from build123d import *

# Parameters (mm, degrees)
F0_R     = 26.289
F0_R_2   = 5.207
F1_DEPTH = 15.24
F2_R     = 28.829
F2_R_2   = 5.207
F3_DEPTH = 2.54
F5_DEPTH = 17.781
F6_COUNT = 3
F6_ANGLE = 240
F8_SIZE2 = 1.27
F8_SIZE  = 0.3402954744


with BuildPart() as f1:
    # F0 (on Right) → F1 (new body)
    with BuildSketch(Plane.YZ):
        Circle(F0_R)
        Circle(F0_R_2, mode=Mode.SUBTRACT)
    extrude(amount=-F1_DEPTH)

    # F2 (on face) → F3 (join)
    with BuildSketch(Plane.YZ):
        Circle(F2_R)
        Circle(F2_R_2, mode=Mode.SUBTRACT)
    extrude(amount=F3_DEPTH)


with BuildPart() as f5:
    # F4 (on face) → F5 (new body, through all)
    with BuildSketch(Plane(origin=(-15.24, 0, 0), x_dir=(0, -1, 0), z_dir=(-1, 0, 0))):
        with BuildLine():
            ThreePointArc((-28.3910227116, -5.006103314), (-23.5858740231, -39.2113912621), (8.8826653964, -27.4264379104))
            add(Edge.make_bspline(
                [(8.8826653964, -27.4264379104), (8.6161177773, -26.6034358722), (8.3394760096, -25.8031213114), (8.0525136679, -25.025358032)],
                knots=[0, 0, 0, 0, 1.8877220202, 1.8877220202, 1.8877220202, 1.8877220202], degree=3))
            ThreePointArc((8.0525136679, -25.025358032), (-13.5505111701, -22.527653407), (-25.8808899077, -4.6142235084))
            add(Edge.make_bspline(
                [(-25.8808899077, -4.6142235084), (-26.7024403228, -4.7252100836), (-27.5390757823, -4.8558820842), (-28.3910227116, -5.006103314)],
                knots=[41.6093954543, 41.6093954543, 41.6093954543, 41.6093954543, 43.4971174745, 43.4971174745, 43.4971174745, 43.4971174745], degree=3))
        make_face()
        with BuildLine():
            ThreePointArc((-25.8808899077, -4.6142235084), (-13.5505111701, -22.527653407), (8.0525136679, -25.025358032))
            add(Edge.make_bspline(
                [(8.0525136679, -25.025358032), (2.0142176142, -8.6595697091), (-8.5937274184, -2.2788306654), (-25.8808899077, -4.6142235084)],
                knots=[1.8877220202, 1.8877220202, 1.8877220202, 1.8877220202, 41.6093954543, 41.6093954543, 41.6093954543, 41.6093954543], degree=3))
        make_face()
    extrude(amount=-F5_DEPTH)


with BuildPart() as f6_1:
    # F6: instance of F5
    add(f5.part.rotate(Axis((0, 0, 0), (1, 0, 0)), 1 * F6_ANGLE / (F6_COUNT - 1)))


with BuildPart() as f6_2:
    # F6: instance of F5
    add(f5.part.rotate(Axis((0, 0, 0), (1, 0, 0)), 2 * F6_ANGLE / (F6_COUNT - 1)))


with BuildPart() as f1_1:
    add(f1.part)

    # F7: cut F5, F6_2, F6_1
    add(f5.part, mode=Mode.SUBTRACT)
    add(f6_2.part, mode=Mode.SUBTRACT)
    add(f6_1.part, mode=Mode.SUBTRACT)

    # F8
    f8_edges = [f1_1.edges().sort_by_distance(p)[0] for p in [
        (-15.24, 26.284776, 0.47126),
        (-15.24, -13.550511, 22.527653),
        (-15.24, -12.734265, -22.998914),
    ]]
    f8_side = f1_1.faces().sort_by_distance((-15.24, 4.091505, 7.389523))[0]
    chamfer(f8_edges, length=F8_SIZE, length2=F8_SIZE2, reference=f8_side)


solid = f1_1.part
Could you check a few things on this model? Use its own coordinates, in mm. A direction names the side the tool comes from. Coordinates: 2 decimals unless noted, no trailing zeros.
1. For faces 1 (the face through (1.3, -14, -25.2)), 2 (the face through (-6.887, -12.797, -22.964)), 3 (the face through (-6.887, -13.489, 22.564)), 4 (the face through (-6.887, 26.286, 0.4)), which set-ups out of +Z, -Z, +X, -X, +Y, -Y let a thin tool reach every point of the face, with its end or its side?
2. I need wall thicknesses on L1, parallel to Z at x = -10.5, y = 0; L2, parallel to Z at x = -13.5, y = -2; L3, parallel to Z at x = -14.25, y = 19. Which ranges of each line are inside material? Lowest first, please.
3. For P1, Ø2, axis at x = -8, y = 22, coming from the -Z side; P2, Ø3, axis at x = -12.5, y = 1, coming from the +Z side; P3, Ø8, axis at x = -10.5, y = 1.5, coming from the -Z side, each with a flat end and sliding along its axis, tell me the tip position at first contact or that it passes through.
4. We'd pull the mould along Z, two halves only. Please class faces 5 (the face through (-6.474, 4.967, 1.564)), 6 (the face through (0, -14, 24)), 7 (the face through (-14.596, 26.118, 0.397)), 8 (the face through (1.252, -14.793, 24.744)): released by +Z, released by -Z, zero draft, split by the parting line, or undercut.
Computed values:
1. face 1: -Z, +X, -X, -Y
1. face 2: -Z, -X, -Y
1. face 3: +Z, -X, -Y
1. face 4: -X, +Y
2. L1: z = -11.51 to -5.21, 5.21 to 11.13
2. L2: z = -13.77 to -4.81, 4.81 to 13.13
2. L3: z = -4.15 to 4.83
3. P1: stops at z = -4.3
3. P2: stops at z = 11.59
3. P3: stops at z = -14.42
4. face 5: undercut
4. face 6: zero draft
4. face 7: split by the parting line
4. face 8: released by +Z
